Part print with two shaded views. Sizes in mm from the minimum x, y, z corner. A direction names the side the tool comes from. Give positions to 0.01 mm unless a question says otherwise; leave off trailing zeros. Write each loop counter-clockwise with the first axis right and the second up, starting at its lowest first coordinate (ties: lowest second). Pieces come first, ordered by that corner, then holes. Notation, with made-up numbers: (-26, 57.25) - (-19, 57.25) arc R24 cw to (-19, 92.25) - close; hole circle Ø9 at (-23.5, -3). An arc over 180 degrees is marked (long way). Answer as a JSON object with one key per item and string values. Group by question number.
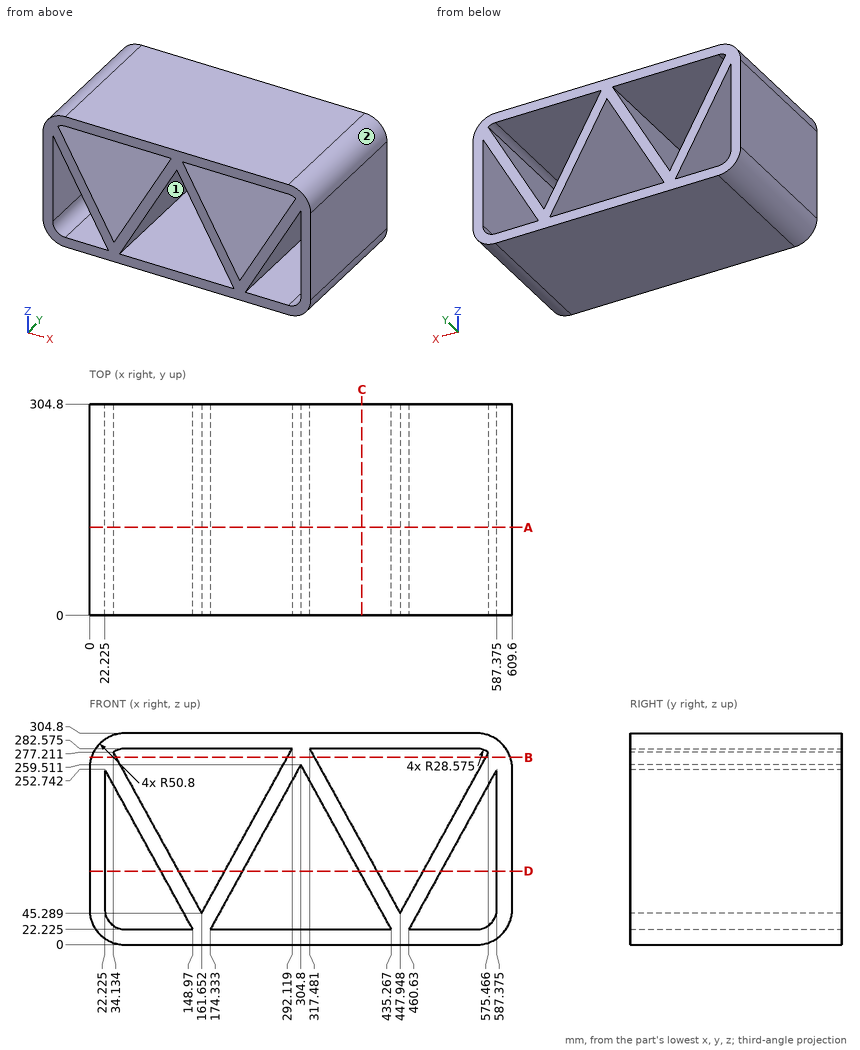
1) Drill centre lines: line 1 along Z through (x, y) = (397.5, 19.5) (1 decimal); line 2 along Z through (x, y) = (280, 289) (1 decimal); line 3 along X through (y, z) = (50, 103) (1 decimal). Where is each one in solid material? Low to high. Write a range as from..to.
2) Saw through at B-B (z = 270). List the corners of the cut face in (x, y) (1 decimal), and give its area (3 significant figures).
3) Saw through at C-C (x = 393). List the corners of the cut face in (y, z) (1 decimal), and give its area (3 significant figures).
4) Drop a flat-ended pin along its axis: P1, Ø12, axis at y = 240.5, z = 35, coming from the -X side (1 decimal). Give the stop position or say it passes through.
5) Saw through at D-D (z = 106). List the corners of the cut face in (x, y) (1 decimal), and give its area (3 significant figures).
6) Which spindle directions (+Z, -Z, +X, -X, +Y, -Y) get a long thin tool onto all of the face, cutting with end or side? Do the marked faces 1 and 2. Say none if no direction does.
7) Saw through at A-A (y = 127). State how many separate pieces and enclosed holes the cut face has, and give its area (3 significant figures).
Checks:
{
 "1": {"line 1": "0..22.2, 90.9..137, 282.6..304.8", "line 2": "0..22.2, 214.4..260.5, 282.6..304.8", "line 3": "0..22.2, 104.6..129.9, 193.4..218.7, 390.9..416.2, 479.7..505, 587.4..609.6"},
 "2": {"outline": "(2.6, 0) - (38.1, 0) - (38.1, 304.8) - (2.6, 304.8) - close; (285.2, 0) - (324.4, 0) - (324.4, 304.8) - (285.2, 304.8) - close; (571.5, 0) - (607, 0) - (607, 304.8) - (571.5, 304.8) - close", "area": "33,600 mm2"},
 "3": {"outline": "(0, 0) - (304.8, 0) - (304.8, 22.2) - (0, 22.2) - close; (0, 99.1) - (304.8, 99.1) - (304.8, 145.2) - (0, 145.2) - close; (0, 282.6) - (304.8, 282.6) - (304.8, 304.8) - (0, 304.8) - close", "area": "27,600 mm2"},
 "4": {"P1": "x = 1"},
 "5": {"outline": "(0, 0) - (22.2, 0) - (22.2, 304.8) - (0, 304.8) - close; (102.9, 0) - (128.3, 0) - (128.3, 304.8) - (102.9, 304.8) - close; (195, 0) - (220.4, 0) - (220.4, 304.8) - (195, 304.8) - close; (389.2, 0) - (414.6, 0) - (414.6, 304.8) - (389.2, 304.8) - close; (481.3, 0) - (506.7, 0) - (506.7, 304.8) - (481.3, 304.8) - close; (587.4, 0) - (609.6, 0) - (609.6, 304.8) - (587.4, 304.8) - close", "area": "44,500 mm2"},
 "6": {"face 1": "+Y, -Y", "face 2": "+Z, +X, +Y, -Y"},
 "7": {"separate pieces": "1", "enclosed holes": "5", "area": "61,900 mm2"}
}
